Can you work these out from the model? Positions are in its coordinate system, mm. Face numbers are marked on the shaded views. Round coordinates to 2 decimals unless told otherwise and drop trailing zeros. Loops run counter-clockwise (first coordinate to the right, second up) from the corner with the lowest first, then second, coordinate; pieces in that order, holes last. Notation, with made-up numbers: M 8.25,37.25 L 50.25,37.25 A16 ccw 50.25,64.25 Z; hole C -20.75,26 d11. An arc over 180 degrees is marked long. Return JSON: item names as keys, results as strings.
Autodesk Inventor part; units mm, degrees
ref_plane "YZ Plane" through (0, 0, 0) normal (1, 0, 0) x (0, 1, 0)
ref_plane "XZ Plane" through (0, 0, 0) normal (0, 1, 0) x (-1, 0, 0)
ref_plane "XY Plane" through (0, 0, 0) normal (0, 0, 1) x (1, 0, 0)
sketch "Sketch1" plane through (0, 0, 0) normal (1, 0, 0) x (0, 1, 0)
  point P0 (0, 0)
sketch "Sketch2" plane through (0, 0, 0) normal (1, 0, 0) x (0, 1, 0)
  circle A0 centre (0, 0) radius 17.5
  circle A1 centre (35.0665, 0.0228) radius 5.5
  circle A2 centre (-17.553, 30.3571) radius 5.5
  circle A3 centre (-17.5135, -30.3799) radius 5.5
  circle A4 centre (-17.5135, -30.3799) radius 12
  circle A5 centre (35.0665, 0.0228) radius 12
  circle A6 centre (-17.553, 30.3571) radius 12
  line L0 (-29.5135, -30.3877) -> (-29.553, 30.3493)
  line L1 (-11.5597, 40.7533) -> (41.0597, 10.419)
  line L2 (41.0732, -10.3656) -> (-11.5068, -40.7683)
  arc A7 (34.6387, -5.4605) -> (34.6316, 5.5056) centre (0, 0) ccw
  arc A8 (-26.717, 22.6098) -> (-29.5455, 18.7634) centre (0, 0) ccw
  arc A9 (-29.521, -18.8018) -> (-26.6876, -22.6445) centre (0, 0) ccw
  arc A10 (31.0434, -16.1651) -> (32.9545, -11.7899) centre (0, 0) ccw
  dimension "d0" = 35
  dimension "d2" = 11
  dimension "d5" = 360
  dimension "d7" = 24
  dimension "d8" = 24
  dimension "d9" = 24
extrude "Extrusion1" add sketch "Sketch2" along normal blind 20
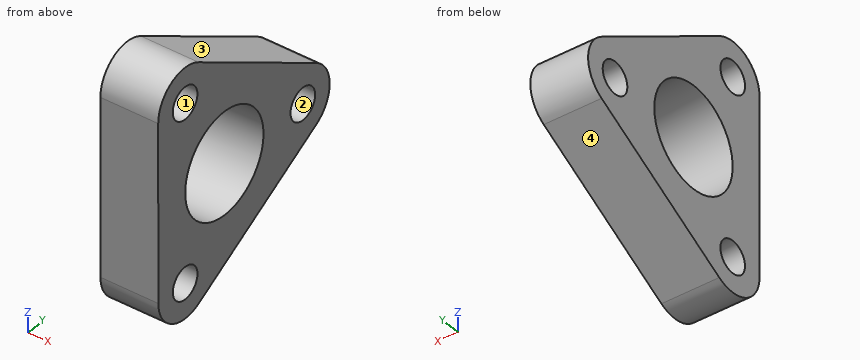
Q1. Suppose I cut it at D-D, the plane z = 19.5. Please give me the cut outline in (x, y).
Results:
{"outline": "M 0,-29.55 L 20,-29.55 L 20,25.31 L 0,25.31 Z"}
Q2. Suppose I cut it at C-C, the plane x = 15.5. Please give me the cut outline in (y, z).
Results:
{"outline": "M -29.55,30.35 L -29.51,-30.39 A12 ccw -11.51,-40.77 L 41.07,-10.37 A12 ccw 41.06,10.42 L -11.56,40.75 A12 ccw Z; hole C -17.55,30.36 d11; hole C -17.51,-30.38 d11; hole C 0,0 d35; hole C 35.07,0.02 d11"}
Q3. Suppose I cut it at B-B, the plane z = -9. Please give me the cut outline in (x, y).
Results:
{"outline": "M 0,-29.53 L 20,-29.53 L 20,-15.01 L 0,-15.01 Z; M 0,15.01 L 20,15.01 L 20,42.98 L 0,42.98 Z"}
Q4. Thinking about a two-plate mould opening in Z: for the marked faces 1, 2, 3 and 4, which applies, pulls with the +Z half, pulls with the -Z half, needs draft (parallel to the pull), parting line crosses it, or undercut?
Results:
{"face 1": "undercut", "face 2": "undercut", "face 3": "pulls with the +Z half", "face 4": "pulls with the -Z half"}
Q5. If I drill on line 1 along Y through (x, z) = (1.75, 0.5); line 2 along Y through (x, z) = (16, 1); line 3 along Y through (x, z) = (5, 7.5), over which ranges is the centre line in solid material (lowest first)?
Results:
{"line 1": "y = -29.53 to -17.49, 17.49 to 29.59, 40.55 to 47.06", "line 2": "y = -29.53 to -17.47, 17.47 to 29.65, 40.48 to 47.03", "line 3": "y = -29.54 to -15.81, 15.81 to 44.45"}
Q6. Suppose I cut it at A-A, the plane y = 34. Please give me the cut outline in (x, z).
Results:
{"outline": "M 0,-14.46 L 20,-14.46 L 20,-5.37 L 0,-5.37 Z; M 0,5.42 L 20,5.42 L 20,14.49 L 0,14.49 Z"}
Q7. I'm going to push flat-ended pins straight in: pin 1 Ø6 at (x, z) = (16.5, -25) entering from -Y; pin 2 Ø1 at (x, y) = (3, 26.5) entering from -Z; pin 3 Ø12 at (x, z) = (15.5, 6.5) entering from +Y. Where does each tip first touch, or does it pass through?
Results:
{"pin 1": "stops at y = -29.52", "pin 2": "stops at z = -19.08", "pin 3": "stops at y = 47.06"}
